```python
from build123d import *

# Parameters (mm, degrees)
BOSS_EXTRUDE1_DEPTH  = 640
BOSS_EXTRUDE2_DEPTH  = 8
BOSS_EXTRUDE3_DEPTH  = 72
SKETCH6_R            = 4
CUT_EXTRUDE1_DEPTH   = 8
FILLET1_R            = 10
FILLET2_R            = 8
FILLET1_OF_MIRROR1_R = 10
FILLET2_OF_MIRROR1_R = 8


with BuildPart() as part:
    # Sketch1 → Boss-Extrude1 (new body)
    with BuildSketch(Plane.XY):
        Polygon((-8, 8), (72, 8), (72, 0), (0, 0), (0, -72), (-8, -72), align=None)
    boss_extrude1 = extrude(amount=BOSS_EXTRUDE1_DEPTH)

    # Sketch3 → Boss-Extrude2 (add)
    with BuildSketch(Plane(origin=(0, 0, 0), x_dir=(1, 0, 0), z_dir=(0, 1, 0))):
        Polygon((-8, -640), (34.5, -713.612159322), (72, -713.612159322), (72, -640), align=None)
    boss_extrude2 = extrude(amount=BOSS_EXTRUDE2_DEPTH)

    # Sketch4 → Boss-Extrude3 (add)
    with BuildSketch(Plane.XZ):
        Polygon((-8, 640), (34.5, 713.612159322), (40.5, 710.148057707), (0, 640), align=None)
    boss_extrude3 = extrude(amount=BOSS_EXTRUDE3_DEPTH)

    # Sketch6 → Cut-Extrude1 (cut)
    with BuildSketch(Plane(origin=(-277.128129211, 0, 160), x_dir=(-0.4999999999999956, 0, -0.8660254037844413), z_dir=(0.8660254037844413, 0, -0.4999999999999956))):
        with Locations((-615.006258422, -18)):
            Circle(SKETCH6_R)
        with Locations((-574.506258422, -18)):
            Circle(SKETCH6_R)
        with Locations((-574.506258422, -54)):
            Circle(SKETCH6_R)
        with Locations((-615.006258422, -54)):
            Circle(SKETCH6_R)
    cut_extrude1 = extrude(amount=-CUT_EXTRUDE1_DEPTH, mode=Mode.SUBTRACT)

    # Fillet1
    fillet1_edges = [part.edges().sort_by_distance(p)[0] for p in [
        (0, -36, 640),
        (-8, -32, 640),
    ]]
    fillet(fillet1_edges, radius=FILLET1_R)

    # Fillet2
    fillet2_edges = [part.edges().sort_by_distance(p)[0] for p in [
        (20.919872981, 0, 676.234282891),
        (0, 0, 318.660254038),
        (0.340741737, 0, 639.908698527),
    ]]
    fillet(fillet2_edges, radius=FILLET2_R)

    # Mirror1: Boss-Extrude1, Boss-Extrude2, Boss-Extrude3, Cut-Extrude1 across plane
    add(boss_extrude1.mirror(Plane.XY))
    add(boss_extrude2.mirror(Plane.XY))
    add(boss_extrude3.mirror(Plane.XY))
    add(cut_extrude1.mirror(Plane.XY), mode=Mode.SUBTRACT)

    # Fillet1 of Mirror1
    fillet1_of_mirror1_edges = [part.edges().sort_by_distance(p)[0] for p in [
        (0, -36, -640),
        (-8, -32, -640),
    ]]
    fillet(fillet1_of_mirror1_edges, radius=FILLET1_OF_MIRROR1_R)

    # Fillet2 of Mirror1
    fillet2_of_mirror1_edges = [part.edges().sort_by_distance(p)[0] for p in [
        (20.919872981, 0, -676.234282891),
        (0, 0, -318.660254038),
        (0.340741737, 0, -639.908698527),
    ]]
    fillet(fillet2_of_mirror1_edges, radius=FILLET2_OF_MIRROR1_R)


solid = part.part
```
Check sheet for the modelled part. Datum: model origin and axes. Units: mm. A direction names the side the tool comes from. Round coordinates to 2 decimals unless told otherwise and drop trailing zeros. Loops run counter-clockwise (first coordinate to the right, second up) from the corner with the lowest first, then second, coordinate; pieces in that order, holes last. Notation, with made-up numbers: (41, 48) - (78, 48) arc R15 cw to (78, 65) - close; hole circle Ø7 at (68.25, 84.25). An arc over 180 degrees is marked (long way). Write item = value, one per line. Start each with the question number.
Q1. Access from +Z, -Z, +X, -X, +Y, -Y to the whole of each face (thin tool, end or side, straight path). Record for faces 1 (the face through (31, 8, 10)), 2 (the face through (21.194, -39.552, -676.709)).
Q2. Section check A-A (y = -38). Record the boundary of the cut face in (x, z), plus the area to 3 significant figures.
Q3. Thickness scan on L1, parallel to Y at x = 50.5, z = -619; L2, parallel to X at y = -22, z = -290.5; L3, parallel to Z at x = 24, y = -4. Record the ranges inside material, lowest first.
Q4. Section check B-B (z = 389.5). Record the boundary of the cut face in (x, y).
Q5. Release check for a two-part mould opening along Z. For faces 3 (the face through (21.194, -39.552, 676.709)), 4 (the face through (13.632, -31.44, -677.467)), 5 (the face through (22.62, -2.41, -674.62)), 6 (the face through (13.632, -31.44, 677.467)) record: pulls with the +Z half, pulls with the -Z half, needs draft (parallel to the pull), parting line crosses it, or undercut.
Q6. Depth check by flat-ended pin: P1, Ø12, axis at y = -17.5, z = -66.5, coming from the +X side; P2, Ø6.5, axis at x = 6, y = -5.5, coming from the -Z side; P3, Ø2, axis at x = 7, z = -304.5, coming from the -Y side. Enter the tip coordinate at first touch or a pass-through.
Derived:
q1.face_1 = +Z, -Z, +X, -X, +Y
q1.face_2 = +X, -Y
q2.outline = (-8, -637.32) arc R10 ccw to (-6.66, -642.32) - (34.5, -713.61) - (40.5, -710.15) - (1.34, -642.32) arc R10 cw to (0, -637.32) - (0, 637.32) arc R10 cw to (1.34, 642.32) - (40.5, 710.15) - (34.5, 713.61) - (-6.66, 642.32) arc R10 ccw to (-8, 637.32) - close
q2.area = 11,400 mm^2
q3.L1 = 0 to 8
q3.L2 = -8 to 0
q3.L3 = -695.43 to -679.43, 679.43 to 695.43
q4.outline = (-8, -72) - (0, -72) - (0, -8) arc R8 cw to (8, 0) - (72, 0) - (72, 8) - (-8, 8) - close
q5.face_3 = undercut
q5.face_4 = pulls with the -Z half
q5.face_5 = undercut
q5.face_6 = pulls with the +Z half
q6.P1 = 0
q6.P2 = -669.88
q6.P3 = -0.25
